from build123d import *

# Parameters (mm, degrees)
SKETCH1_W           = 25.4
SKETCH1_H           = 35.56
SKETCH1_R           = 1.5875
BOSS_EXTRUDE1_DEPTH = 3.175
SKETCH7_W           = 25.4
SKETCH7_H           = 2.54
SKETCH7_H_2         = 7.62
BOSS_EXTRUDE3_DEPTH = 20.32
SKETCH11_R          = 1.5875
CUT_EXTRUDE1_DEPTH  = 10
CHAMFER2_SIZE       = 1.27
SKETCH13_R          = 3.175
CUT_EXTRUDE2_DEPTH  = 12.7
SKETCH14_R          = 7.14375
CUT_EXTRUDE3_DEPTH  = 3.302
CUT_EXTRUDE4_START  = -3.302
SKETCH15_R          = 7.14375
CUT_EXTRUDE4_DEPTH  = 3.302
CUT_EXTRUDE5_DEPTH  = 12.7
SKETCH17_W          = 2.029010409
SKETCH17_H          = 25.4
BOSS_EXTRUDE4_DEPTH = 12.7
CUT_EXTRUDE6_DEPTH  = 46.281333074
SKETCH19_W          = 7.112
SKETCH19_H          = 5.08
CUT_EXTRUDE7_DEPTH  = 45.472672789


with BuildPart() as part:
    # Sketch1 → Boss-Extrude1 (new body)
    with BuildSketch(Plane.XY):
        with Locations((0, 11.43)):
            Rectangle(SKETCH1_W, SKETCH1_H)
        with Locations((-6.35, 2.54)):
            Circle(SKETCH1_R, mode=Mode.SUBTRACT)
        with Locations(Location((6.35, 2.54, 0), (0, 0, 180))):
            Circle(SKETCH1_R, mode=Mode.SUBTRACT)
        with Locations((6.35, 17.78)):
            Circle(SKETCH1_R, mode=Mode.SUBTRACT)
        with Locations(Location((-6.35, 17.78, 0), (0, 0, 180))):
            Circle(SKETCH1_R, mode=Mode.SUBTRACT)
    extrude(amount=BOSS_EXTRUDE1_DEPTH)

    # Sketch7 → Boss-Extrude3 (add)
    with BuildSketch(Plane.XY.offset(3.175)):
        with Locations((0, -5.08)):
            Rectangle(SKETCH7_W, SKETCH7_H)
        with Locations((0, 25.4)):
            Rectangle(SKETCH7_W, SKETCH7_H_2)
    extrude(amount=BOSS_EXTRUDE3_DEPTH)

    # Sketch11 → Cut-Extrude1 (cut)
    with BuildSketch(Plane.XZ.offset(6.35)):
        with BuildLine():
            Line((-3.81, 13.805952441), (-3.814692285, 12.218981082))
            ThreePointArc((-3.814692285, 12.218981082), (0, 8.404288797), (3.814692285, 12.218981082))
            Line((3.814692285, 12.218981082), (3.81, 13.805952441))
            Line((3.81, 13.805952441), (3.81, 17.615952441))
            ThreePointArc((3.81, 17.615952441), (9.167172212, 19.841012117), (12.7, 15.24))
            Line((12.7, 15.24), (12.7, 23.495))
            Line((12.7, 23.495), (-12.7, 23.495))
            Line((-12.7, 23.495), (-12.7, 15.24))
            ThreePointArc((-12.7, 15.24), (-9.167172212, 19.841012117), (-3.81, 17.615952441))
            Line((-3.81, 17.615952441), (-3.81, 13.805952441))
        make_face()
        with Locations((-7.9375, 15.24)):
            Circle(SKETCH11_R)
        with Locations((7.9375, 15.24)):
            Circle(SKETCH11_R)
    extrude(amount=-CUT_EXTRUDE1_DEPTH, mode=Mode.SUBTRACT)

    # Chamfer2
    chamfer2_edges = [part.edges().sort_by_distance(p)[0] for p in [
        (-9.525, -6.35, 15.24),
        (6.35, -6.35, 15.24),
    ]]
    chamfer(chamfer2_edges, length=CHAMFER2_SIZE)

    # Sketch13 → Cut-Extrude2 (cut)
    with BuildSketch(Plane(origin=(0, 29.21, 0), x_dir=(1, 0, 0), z_dir=(0, 1, 0))):
        with Locations(Location((0, -15.24, 0), (0, 0, 270))):
            Circle(SKETCH13_R)
    extrude(amount=-CUT_EXTRUDE2_DEPTH, mode=Mode.SUBTRACT)

    # Sketch14 → Cut-Extrude3 (cut)
    with BuildSketch(Plane(origin=(0, 29.21, 0), x_dir=(1, 0, 0), z_dir=(0, 1, 0))):
        with Locations(Location((0, -15.24, 0), (0, 0, 270))):
            Circle(SKETCH14_R)
    extrude(amount=-CUT_EXTRUDE3_DEPTH, mode=Mode.SUBTRACT)

    # Sketch15 → Cut-Extrude4 (cut)
    with BuildSketch(Plane.XZ.offset(-21.59).offset(CUT_EXTRUDE4_START)):
        with Locations(Location((0, 15.24, 0), (0, 0, 90))):
            Circle(SKETCH15_R)
    extrude(amount=CUT_EXTRUDE4_DEPTH, mode=Mode.SUBTRACT)

    # Sketch16 → Cut-Extrude5 (cut)
    with BuildSketch(Plane(origin=(0, 29.21, 0), x_dir=(1, 0, 0), z_dir=(0, 1, 0))):
        with BuildLine():
            ThreePointArc((8.255, -15.24), (5.837166479, -21.077166479), (0, -23.495))
            Line((0, -23.495), (12.7, -23.495))
            Line((12.7, -23.495), (12.7, -7.184415797))
            ThreePointArc((12.7, -7.184415797), (9.556910358, -8.486326154), (8.255, -11.629415797))
            Line((8.255, -11.629415797), (8.255, -15.24))
        make_face()
        with BuildLine():
            ThreePointArc((0, -23.495), (-5.837166479, -21.077166479), (-8.255, -15.24))
            Line((-8.255, -15.24), (-8.255, -11.629415797))
            ThreePointArc((-8.255, -11.629415797), (-9.556910358, -8.486326154), (-12.7, -7.184415797))
            Line((-12.7, -7.184415797), (-12.7, -23.495))
            Line((-12.7, -23.495), (0, -23.495))
        make_face()
    extrude(amount=-CUT_EXTRUDE5_DEPTH, mode=Mode.SUBTRACT)

    # Sketch17 → Boss-Extrude4 (add)
    with BuildSketch(Plane.XY.offset(3.175)):
        with Locations((-11.685494796, 8.89)):
            Rectangle(SKETCH17_W, SKETCH17_H)
        with Locations((11.685494796, 8.89)):
            Rectangle(SKETCH17_W, SKETCH17_H)
    extrude(amount=BOSS_EXTRUDE4_DEPTH)

    # Sketch18 → Cut-Extrude6 (cut, through all)
    with BuildSketch(Plane(origin=(12.7, 0, 0), x_dir=(0, 0, -1), z_dir=(1, 0, 0))):
        with BuildLine():
            ThreePointArc((-7.184415797, 21.59), (-5.951695656, 7.221633885), (-15.24, -3.81))
            Line((-15.24, -3.81), (-15.875, -3.81))
            Line((-15.875, -3.81), (-15.875, 21.59))
            Line((-15.875, 21.59), (-7.184415797, 21.59))
        make_face()
    extrude(amount=-CUT_EXTRUDE6_DEPTH, mode=Mode.SUBTRACT)

    # Sketch19 → Cut-Extrude7 (cut, through all)
    with BuildSketch(Plane(origin=(0, 29.21, 0), x_dir=(1, 0, 0), z_dir=(0, 1, 0))):
        with Locations((0, -2.54)):
            Rectangle(SKETCH19_W, SKETCH19_H)
    extrude(amount=-CUT_EXTRUDE7_DEPTH, mode=Mode.SUBTRACT)


solid = part.part
Verification items for the finished model (mm, model axes). A direction names the side the tool comes from. Give positions to 0.01 mm unless a question says otherwise; leave off trailing zeros. Order: outer loops, then holes, each group sorted by start corner. A loop starts at its lowest first (then second) coordinate and runs counter-clockwise, first axis right, second up. Notation, with made-up numbers: M 79.25,87 L 129.25,87 A37 cw 129.25,123 Z; hole C 69,15 d3. An arc over 180 degrees is marked long. Use one line per item in the form item = value. Start each with the question number.
Q1. Mould release check, pull along Y, two halves, no side actions. Record for faces 4 (the cylindrical face through (-2.736, 27.582, 21.839)), 5 (the flat face through (-10.671, 6, 5)): +Y half, -Y half, draft (parallel to the pull), parting line (faces both ways), or undercut.
Q2. Go/stop test with flat-tipped pins: pin 1 Ø1.5 at (x, z) = (1, 11) entering from +Y; pin 2 Ø2 at (x, y) = (2.5, 22) entering from -Z; pin 3 Ø1 at (y, z) = (25.5, 19) entering from -X. Record where each tip stops, or that it passes through.
Q3. Section check C-C (y = -3). Enter the section's corners in (x, z) (3 decimals), then the cut area to 3 significant figures.
Q4. Section check D-D (z = 6.25). Enter the section's corners in (x, y).
Q5. Scan lines: line 1 along X through (y, z) = (24.1, 15.24) (3 decimals); line 2 along X through (y, z) = (5.5, 4.5); line 3 along Y through (x, z) = (3, 5.25). Record each from-to range of solid material in increasing order. Write a range as [from, to].
Q6. Section check B-B (z = 10.25). Enter the section's corners in (x, y), then the cut area to 3 significant figures.
Q7. Access from +Z, -Z, +X, -X, +Y, -Y to the whole of each face (thin tool, end or side, straight path). Record for faces 1 (the flat face through (-3, -3.81, 9.6)), 2 (the cylindrical face through (-9.523, 25.453, 8.521)), 3 (the flat face through (0, 25, 5.08)).
Q8. Section check A-A (y = 22). Enter the section's corners in (x, z) (1 decimal).
Evaluation:
q1.face_4 = draft
q1.face_5 = undercut
q2.pin_1 = 25.91
q2.pin_2 = 5.08
q2.pin_3 = -7.58
q3.outline = M -12.7,0 L -3.556,0 L -3.556,3.175 L -10.671,3.175 L -10.671,13.83 L -12.7,13.83 Z; M 3.556,0 L 12.7,0 L 12.7,13.83 L 10.671,13.83 L 10.671,3.175 L 3.556,3.175 Z
q3.area = 101 mm2
q4.outline = M -12.7,-6.35 L 12.7,-6.35 L 12.7,6.35 L 10.67,6.35 L 10.67,-3.81 L -10.67,-3.81 L -10.67,6.35 L -12.7,6.35 Z; M -12.7,19.48 L -10.67,19.48 L -10.67,21.59 L 10.67,21.59 L 10.67,19.48 L 12.7,19.48 L 12.7,29.21 L -12.7,29.21 Z
q5.line_1 = [-8.255, -7.144], [7.144, 8.255]
q5.line_2 = [-12.7, -10.67], [10.67, 12.7]
q5.line_3 = [-6.35, -3.81], [21.59, 29.21]
q6.outline = M -12.7,-6.35 L -3.27,-6.35 L -3.27,-3.81 L -10.67,-3.81 L -10.67,-0.06 L -12.7,-0.06 Z; M -8.47,21.59 L -5.11,21.59 L -5.11,24.89 L 5.11,24.89 L 5.11,21.59 L 8.47,21.59 L 8.47,29.21 L 5.11,29.21 L 5.11,25.91 L -5.11,25.91 L -5.11,29.21 L -8.47,29.21 Z; M 3.27,-6.35 L 12.7,-6.35 L 12.7,-0.06 L 10.67,-0.06 L 10.67,-3.81 L 3.27,-3.81 Z
q6.area = 125 mm2
q7.face_1 = +Z
q7.face_2 = +Z, -X, +Y
q7.face_3 = -Z, +Y, -Y
q8.outline = M -12.7,0 L -3.6,0 L -3.6,5.1 L 3.6,5.1 L 3.6,0 L 12.7,0 L 12.7,7.2 A4.4 cw 8.3,11.6 L 8.3,15.2 A8.3 ccw -8.3,15.2 L -8.3,11.6 A4.4 cw -12.7,7.2 Z; hole C 0,15.2 d14.3
